Can you work these out from the model? Positions are in its coordinate system, mm. Face numbers are marked on the shaded views. A direction names the side the tool comes from. Give positions to 0.01 mm unless a question says otherwise; leave off trailing zeros. Loops run counter-clockwise (first coordinate to the right, second up) from the corner with the lowest first, then second, coordinate; pieces in that order, holes last. Notation, with made-up numbers: (31, -25) - (58, -25) arc R24 ccw to (58, 0) - close; hole circle Ø3 at (-20, 36.25). An arc over 180 degrees is marked (long way). Answer as a JSON object with one key per item and string values.
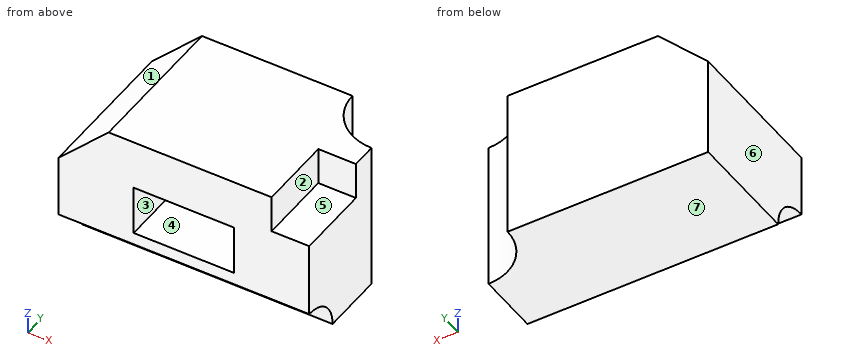
```python
from build123d import *

# Parameters (mm, degrees)
F0_W      = 50
F0_H      = 30
F1_DEPTH  = 30
F3_DEPTH  = 30.001
F4_W      = 20
F4_H      = 10
F5_DEPTH  = 20
F6_R      = 10
F7_DEPTH  = 30.001
F8_W      = 7.5
F8_H      = 15
F9_DEPTH  = 7.5
F10_R     = 7.5
F11_DEPTH = 50.001


with BuildPart() as f1:
    # F0 (on Top) → F1 (new body)
    with BuildSketch(Plane.XY):
        with Locations((25, 15)):
            Rectangle(F0_W, F0_H)
    extrude(amount=F1_DEPTH)

    # F2 (on face) → F3 (cut, through all)
    with BuildSketch(Plane.XZ):
        Polygon((10, 30), (0, 30), (0, 20), align=None)
    extrude(amount=-F3_DEPTH, mode=Mode.SUBTRACT)

    # F4 (on face) → F5 (cut)
    with BuildSketch(Plane.XZ):
        with Locations((25, 15)):
            Rectangle(F4_W, F4_H)
    extrude(amount=-F5_DEPTH, mode=Mode.SUBTRACT)

    # F6 (on face) → F7 (cut, through all)
    with BuildSketch(Plane.XY.offset(30)):
        with Locations((50, 30)):
            Circle(F6_R)
    extrude(amount=-F7_DEPTH, mode=Mode.SUBTRACT)

    # F8 (on face) → F9 (cut)
    with BuildSketch(Plane.XY.offset(30)):
        with Locations((46.25, 7.5)):
            Rectangle(F8_W, F8_H)
    extrude(amount=-F9_DEPTH, mode=Mode.SUBTRACT)

    # F10 (on face) → F11 (cut, through all)
    with BuildSketch(Plane.YZ.offset(50)):
        Circle(F10_R)
    extrude(amount=-F11_DEPTH, mode=Mode.SUBTRACT)


solid = f1.part
```
1) I need wall thicknesses on L1, parallel to X at y = 3.5, z = 16.75; L2, parallel to Z at x = 21, y = 14.5; L3, parallel to Y at x = 19, z = 17.75. Which ranges of each line are inside material? Lowest first, please.
Check sheet entries:
{"L1": "0 to 15, 35 to 50", "L2": "0 to 10, 20 to 30", "L3": "20 to 30"}
2) If we mould it in two halves opening along Z, with no side actions, what happens to the marked faces 4, 5, 6 and 7? For each: released by +Z, released by -Z, zero draft, split by the parting line, or undercut.
Check sheet entries:
{"face 4": "undercut", "face 5": "released by +Z", "face 6": "zero draft", "face 7": "released by -Z"}
3) Imagine slicing it at D-D on y = 3.5. Write out the boundary of the cut face in (x, z).
Check sheet entries:
{"outline": "(0, 6.63) - (50, 6.63) - (50, 22.5) - (42.5, 22.5) - (42.5, 30) - (10, 30) - (0, 20) - close; hole (15, 10) - (35, 10) - (35, 20) - (15, 20) - close"}
4) Imagine slicing it at C-C on x = 23. Write out the boundary of the cut face in (y, z), and give its area (3 significant figures).
Check sheet entries:
{"outline": "(0, 7.5) arc R7.5 cw to (7.5, 0) - (30, 0) - (30, 30) - (0, 30) - (0, 20) - (20, 20) - (20, 10) - (0, 10) - close", "area": "656 mm2"}
5) Imagine slicing it at B-B on z = 13.5. Write out the boundary of the cut face in (x, y).
Check sheet entries:
{"outline": "(0, 0) - (15, 0) - (15, 20) - (35, 20) - (35, 0) - (50, 0) - (50, 20) arc R10 cw to (40, 30) - (0, 30) - close"}
6) I'm going to push flat-ended pins straight in: P1, Ø5, axis at x = 24.5, z = 17, coming from the -Y side; P2, Ø2, axis at y = 10.5, z = 26, coming from the +X side; P3, Ø4, axis at x = 46.5, y = 8.5, coming from the +Z side. Where does each tip first touch, or does it pass through?
Check sheet entries:
{"P1": "y = 20", "P2": "x = 42.5", "P3": "z = 22.5"}
7) Imagine slicing it at A-A on y = 17.5. Write out the boundary of the cut face in (x, z).
Check sheet entries:
{"outline": "(0, 0) - (50, 0) - (50, 30) - (10, 30) - (0, 20) - close; hole (15, 10) - (35, 10) - (35, 20) - (15, 20) - close"}
8) Which directions (+Z, -Z, +X, -X, +Y, -Y) give clear straight access to the entire face, cutting with the end or side of a thin tool? Please do the marked faces 1, 2 and 3.
Check sheet entries:
{"face 1": "+Z, -X, +Y, -Y", "face 2": "+Z, +X, -Y", "face 3": "-Y"}
